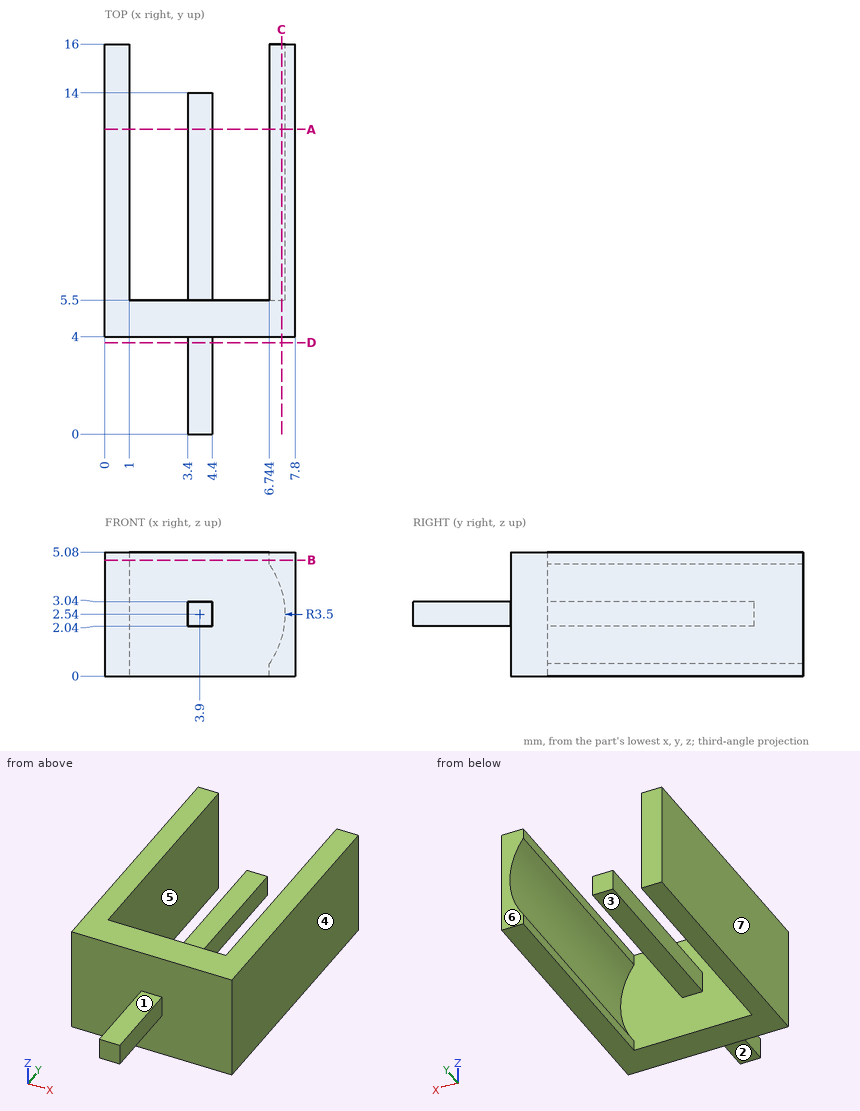
The figure shows three views and two pictorial views of one solid part (mm, origin at its lowest corner). Answer the questions. A direction names the side the tool comes from. Round coordinates to 2 decimals unless told otherwise and drop trailing zeros. Loops run counter-clockwise (first coordinate to the right, second up) from the corner with the lowest first, then second, coordinate; pieces in that order, holes last. Notation, with made-up numbers: M -12.75,-38 L 10.25,-38 A20 cw 10.25,-34 Z; hole C -12,75.25 d11. An arc over 180 degrees is marked long. Write each question's results on one line, items separated by ' | '. Start each with the question number.
1) Each of these flat-tipped pins is pushed along its axis until it touches: pin 1 (1.1 mm diameter, centred on x = 4, z = 2.5, fed in from +Y); pin 2 (1.1 mm diameter, centred on x = 4, y = 1.5, fed in from -Z); pin 3 (0.8 mm diameter, centred on x = 4, y = 2.5, fed in from +Z). Where does it stop, or does it pass through?
2) Find section C-C on x = 7.25. Write down the section's boundary in (y, z), plus the area to 3 significant figures.
3) Straight lines are drawn through the part: probe 1 along X at (y, z) = (12, 2.7); probe 2 along Y at (x, z) = (4.5, 2.1); probe 3 along Y at (x, z) = (0.75, 4.4). For each, find the intervals that lie inside material, in ascending order.
4) Find section A-A on y = 12.5. Write down the section's boundary in (x, z).
5) Find section B-B on z = 4.75. Write down the section's boundary in (x, y).
6) Find section D-D on y = 3.75. Write down the section's boundary in (x, z), plus the area to 3 significant figures.
7) Which of the six approach directions +Z, -Z, +X, -X, +Y, -Y give full straight-line access (tool end or side, diameter ignored) to the marked faces 1, 2 and 3?
8) Determine the mould class of the marked faces 4, 5, 6 and 7 for opening direction X: pulls with the +X half, pulls with the -X half, needs draft (parallel to the pull), parting line crosses it, or undercut.
Final values:
1) pin 1: y = 14 | pin 2: z = 2.04 | pin 3: z = 3.04
2) outline: M 4,0 L 16,0 L 16,1.53 L 5.5,1.53 L 5.5,3.55 L 16,3.55 L 16,5.08 L 4,5.08 Z | area: 39.7 mm²
3) probe 1: 0 to 1, 3.4 to 4.4, 7.4 to 7.8 | probe 2: 4 to 5.5 | probe 3: 4 to 16
4) outline: M 0,0 L 1,0 L 1,5.08 L 0,5.08 Z; M 3.4,2.04 L 4.4,2.04 L 4.4,3.04 L 3.4,3.04 Z; M 6.74,0 L 7.8,0 L 7.8,5.08 L 6.74,5.08 L 6.74,4.58 A3.5 cw 6.74,0.5 Z
5) outline: M 0,4 L 7.8,4 L 7.8,16 L 6.74,16 L 6.74,5.5 L 1,5.5 L 1,16 L 0,16 Z
6) outline: M 3.4,2.04 L 4.4,2.04 L 4.4,3.04 L 3.4,3.04 Z | area: 1.00 mm²
7) face 1: +Z, +X, -X, -Y | face 2: -Z, +X, -X, -Y | face 3: -Z, +Y
8) face 4: pulls with the +X half | face 5: undercut | face 6: needs draft | face 7: pulls with the -X half
